For this review, take the finished solid that the model builds, in its own axes (mm). Round coordinates to 2 decimals unless told otherwise and drop trailing zeros. Write each loop counter-clockwise with the first axis right and the second up, starting at its lowest first coordinate (ties: lowest second). Pieces come first, ordered by that corner, then holes.
Autodesk Inventor part; units mm, degrees
ref_plane "YZ Plane" through (0, 0, 0) normal (1, 0, 0) x (0, 1, 0)
ref_plane "XZ Plane" through (0, 0, 0) normal (0, 1, 0) x (-1, 0, 0)
ref_plane "XY Plane" through (0, 0, 0) normal (0, 0, 1) x (1, 0, 0)
sketch "Sketch1" plane through (0, 0, 0) normal (1, 0, 0) x (0, 1, 0)
  line L0 (0, 0) -> (609.6, 0)
  line L1 (609.6, 0) -> (609.6, -50.8)
  line L2 (609.6, -50.8) -> (0, -50.8)
  line L3 (0, -50.8) -> (0, 0)
  circle A0 centre (8.89, -25.4) radius 11.049
  circle A1 centre (8.89, -7.62) radius 2
  circle A2 centre (8.89, -43.18) radius 2
  circle A3 centre (596.9, -12.7) radius 2
  circle A4 centre (596.9, -38.1) radius 2
  circle A5 centre (571.5, -12.7) radius 2
  circle A6 centre (571.5, -38.1) radius 2
  point P0 (0, -25.4)
  point P1 (0, -18.8389)
  point P2 (0, -31.9611)
  dimension "d0" = 609.6
  dimension "d1" = 50.8
  dimension "d2" = 22.098
  dimension "d3" = 8.89
  dimension "d4" = 4
  dimension "d5" = 4
  dimension "d6" = 7.62
  dimension "d7" = 8.89
  dimension "d8" = 7.62
  dimension "d9" = 8.89
  dimension "d10" = 4
  dimension "d11" = 4
  dimension "d12" = 4
  dimension "d13" = 4
  dimension "d14" = 25.4
  dimension "d15" = 25.4
  dimension "d16" = 25.4
  dimension "d17" = 25.4
  dimension "d18" = 12.7
  dimension "d19" = 12.7
extrude "Extrusion1" add sketch "Sketch1" along normal blind 3 contours L0 L1 L2 L3 A0
fillet "Fillet1" radius 6.35 4 edges at (1.5, 0, -31.9611) (1.5, 0, -18.8389) (1.5, 0, 0) (1.5, 0, -50.8)
properties part number "DropBar"
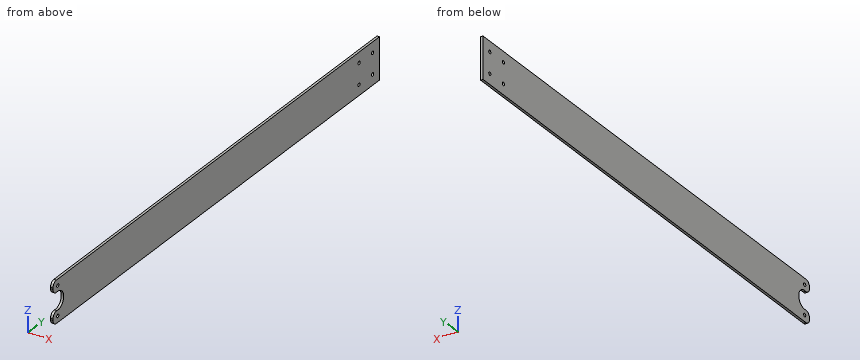
(1) We need section B-B, the plane z = -24.5. Give the boundary of the cut face in (x, y).
Geometry check:
outline: (0, 19.9) - (3, 19.9) - (3, 609.6) - (0, 609.6) - close
(2) For line 1 along Z through (x, y) = (1.9, 8.89); line 2 along Y through (x, z) = (0.5, -7); line 3 along Y through (x, z) = (0.75, -42), list the stretches that pass through material, from the lowest coordinate up.
Geometry check:
line 1: z = -50.8 to -45.18, -41.18 to -36.45, -14.35 to -9.62, -5.62 to 0
line 2: y = 0 to 6.99, 10.79 to 609.6
line 3: y = 0.03 to 7.28, 10.5 to 609.6
(3) We need section A-A, the plane x = 2.1. Give the boundary of the cut face in (y, z).
Geometry check:
outline: (0, -44.45) arc R6.35 ccw to (6.35, -50.8) - (609.6, -50.8) - (609.6, 0) - (6.35, 0) arc R6.35 ccw to (0, -6.35) - (0, -8.19) arc R6.35 ccw to (7.28, -14.47) arc R11.05 cw (long way) to (7.28, -36.33) arc R6.35 ccw to (0, -42.61) - close; hole circle Ø4 at (8.89, -43.18); hole circle Ø4 at (8.89, -7.62); hole circle Ø4 at (571.5, -38.1); hole circle Ø4 at (571.5, -12.7); hole circle Ø4 at (596.9, -38.1); hole circle Ø4 at (596.9, -12.7)
